Answer from the drawing. Dimensions are ordinates in mm from the lowest x, y and z of the part. Round coordinates to 2 decimals unless told otherwise and drop trailing zeros. Order: outer loops, then holes, each group sorted by start corner. A loop starts at its lowest first (then second) coordinate and runs counter-clockwise, first axis right, second up. Notation, with made-up numbers: (74.25, -1.75) -> (133.25, -1.75) arc R14 ccw to (133.25, 25.25) -> close; hole circle Ø9 at (66.25, 49). An arc over 180 degrees is marked (long way). Use a Markdown table: item, result. Add a question column.
1. Given pin 1 (0.9 mm diameter, centred on x = 67.5, z = 1.5, fed in from -Y); pin 2 (1.5 mm diameter, centred on y = 80.5, z = 1, fed in from +X), each flat-ended and moving along its own axis, determine where each tip first touches the part or whether it passes through.
2. Section B-B, the plane z = 1.5 is taken. Give the vertices of the cut face in (x, y), then the cut area to 4 significant figures.
3. Section A-A, the plane x = 84 is taken. Give the vertices of the cut face in (y, z).
4. Section C-C, the plane y = 52.5 is taken. Give the vertices of the cut face in (x, z), then the cut area to 3 significant figures.
5. Consider L1, parallel to Y at x = 84, z = 1.2; L2, parallel to X at y = 62.5, z = 2.9. Determine where each line is inside the solid, lowest interval first. Write a range as [from, to].
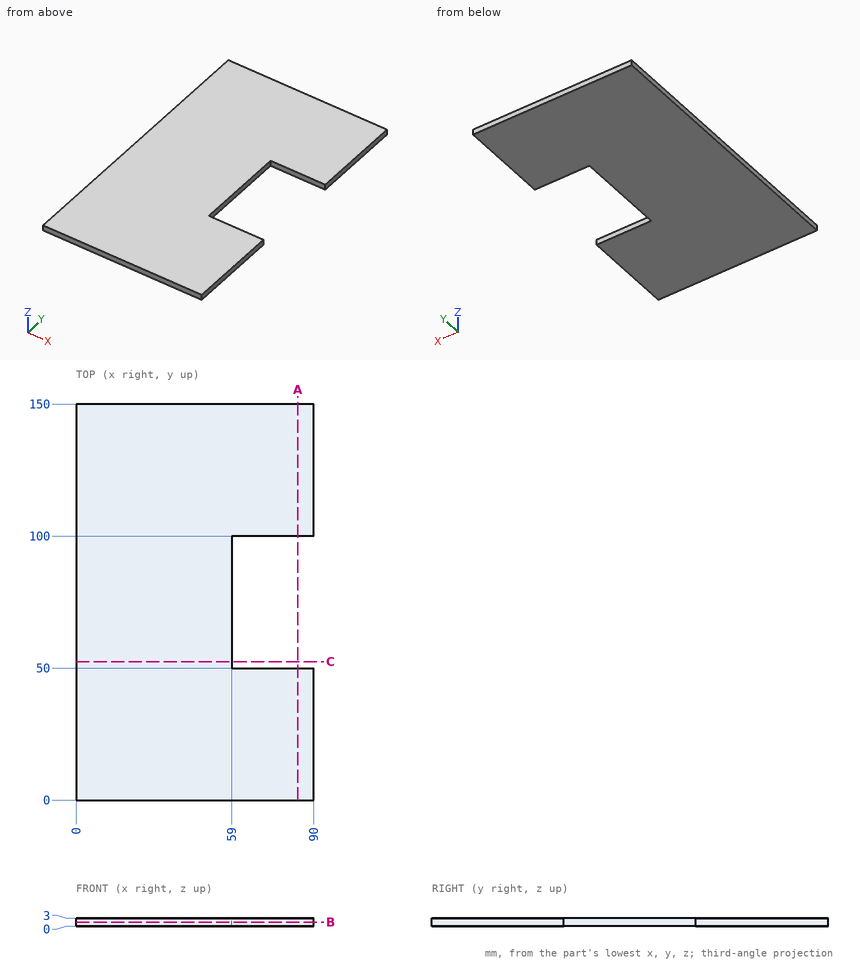
Verdict:
| question | item | result |
|---|---|---|
| 1 | pin 1 | stops at y = 0 |
| 1 | pin 2 | stops at x = 59 |
| 2 | outline | (0, 0) -> (90, 0) -> (90, 50) -> (59, 50) -> (59, 100) -> (90, 100) -> (90, 150) -> (0, 150) -> close |
| 2 | area | 11,950 mm2 |
| 3 | outline | (0, 0) -> (50, 0) -> (50, 3) -> (0, 3) -> close; (100, 0) -> (150, 0) -> (150, 3) -> (100, 3) -> close |
| 4 | outline | (0, 0) -> (59, 0) -> (59, 3) -> (0, 3) -> close |
| 4 | area | 177 mm2 |
| 5 | L1 | y = [0, 50], [100, 150] |
| 5 | L2 | x = [0, 59] |
